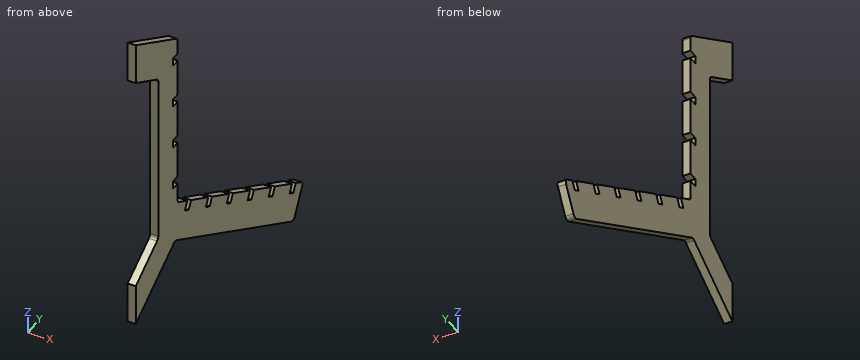
```python
from build123d import *

# Parameters (mm, degrees)
ESTRUSIONE_ESTRUSIONE1_DEPTH = 18
RACCORDO1_R                  = 10
RACCORDO2_R                  = 10


with BuildPart() as part:
    # Schizzo1 → Estrusione-Estrusione1 (new body)
    with BuildSketch(Plane(origin=(0, 0, 0), x_dir=(0, 0, -1), z_dir=(1, 0, 0))):
        Polygon((-109.503770047, 350), (-109.503770047, 330), (-127.503770047, 330), (-127.503770047, 350), (-209.503770047, 350), (-209.503770047, 330), (-227.503770047, 330), (-227.503770047, 350), (-309.503770047, 350), (-309.503770047, 330), (-327.503770047, 330), (-327.503770047, 350), (-363.727557783, 350), (-463.727557783, 176.794919243), (-371.351514713, 176.794919243), (-317.539536248, 270), (70.913458368, 270), (124.725436833, 176.794919243), (217.101479903, 176.794919243), (122.874982595, 340), (405.554474519, 829.615242271), (336.272442217, 869.615242271), (318.31248319, 838.507680735), (335.632991266, 828.507680735), (326.632991266, 812.919223467), (309.31248319, 822.919223467), (268.31248319, 751.905140356), (285.632991266, 741.905140356), (276.632991266, 726.316683088), (259.31248319, 736.316683088), (218.31248319, 665.302599978), (235.632991266, 655.302599978), (226.632991266, 639.71414271), (209.31248319, 649.71414271), (168.31248319, 578.7000596), (185.632991266, 568.7000596), (176.632991266, 553.111602331), (159.31248319, 563.111602331), (118.31248319, 492.097519221), (135.632991266, 482.097519221), (126.632991266, 466.509061953), (109.31248319, 476.509061953), (68.31248319, 405.494978843), (85.632991266, 395.494978843), (76.632991266, 379.906521574), (59.31248319, 389.906521574), (36.272442217, 350), (-9.503770047, 350), (-9.503770047, 330), (-27.503770047, 330), (-27.503770047, 350), align=None)
    extrude(amount=ESTRUSIONE_ESTRUSIONE1_DEPTH)

    # Raccordo1
    raccordo1_edges = [part.edges().sort_by_distance(p)[0] for p in [
        (9, 350, -36.272442217),
    ]]
    fillet(raccordo1_edges, radius=RACCORDO1_R)

    # Raccordo2
    raccordo2_edges = [part.edges().sort_by_distance(p)[0] for p in [
        (9, 869.615242271, -336.272442217),
        (9, 829.615242271, -405.554474519),
        (9, 340, -122.874982595),
        (9, 270, -70.913458368),
        (9, 270, 317.539536248),
        (9, 350, 363.727557783),
    ]]
    fillet(raccordo2_edges, radius=RACCORDO2_R)


solid = part.part
```
Input: part model. Units: mm. Frame: model coordinates. Coordinates: 2 decimals unless noted, no trailing zeros. Loops run counter-clockwise (first coordinate to the right, second up) from the corner with the lowest first, then second, coordinate; pieces in that order, holes last. Notation, with made-up numbers: (-6.5, -30) - (41.5, -30) arc R19 ccw to (41.5, 0) - close; hole circle Ø7 at (-31.5, -23.5). An arc over 180 degrees is marked (long way). Answer in a Markdown table with one row per item.
(1) Cut plane A-A on y = 232. Output: boundary loops of the cut face in (x, z), plus the area to 3 significant figures.
Model answer:
| item | result |
|---|---|
| outline | (0, -185.23) - (18, -185.23) - (18, -92.85) - (0, -92.85) - close; (0, 339.48) - (18, 339.48) - (18, 431.85) - (0, 431.85) - close |
| area | 3,330 mm² |
(2) Material intervals for L1, parallel to Z at x = 8.5, y = 331.5; L2, parallel to Z at x = 11.5, y = 349; L3, parallel to Y at x = 16, z = -153, sorted ascending. Write a range as from..to.
Model answer:
| item | result |
|---|---|
| L1 | z = -127.78..9.5, 27.5..109.5, 127.5..209.5, 227.5..309.5, 327.5..374.41 |
| L2 | z = -128.07..9.5, 27.5..109.5, 127.5..209.5, 227.5..309.5, 327.5..362.31 |
| L3 | y = 176.79..287.82, 392.18..552.18 |
(3) Cut plane B-B on y = 774. Output: boundary loops of the cut face in (x, z) (3 decimals).
Model answer:
| item | result |
|---|---|
| outline | (0, -373.445) - (18, -373.445) - (18, -281.069) - (0, -281.069) - close |
(4) Cut plane C-C on z = 408. Output: boundary loops of the cut face in (x, y), plus the area to 3 significant figures.
Model answer:
| item | result |
|---|---|
| outline | (0, 176.79) - (18, 176.79) - (18, 273.32) - (0, 273.32) - close |
| area | 1,740 mm² |
(5) Pin query (flat end, axial travel): P1, Ø5.5, axis at x = 12.5, z = 182, coming from the +Y side; P2, Ø2, axis at x = 2, z = -248.5, coming from the +Y side; P3, Ø5.5, axis at x = 10.5, y = 336, coming from the -Z side; P4, Ø6, axis at y = 549, z = -240, coming from the -X side. Return the tip coordinate at first contact, or that it passes through.
Model answer:
| item | result |
|---|---|
| P1 | stops at y = 350 |
| P2 | stops at y = 719.32 |
| P3 | stops at z = -126.77 |
| P4 | stops at x = 0 |
